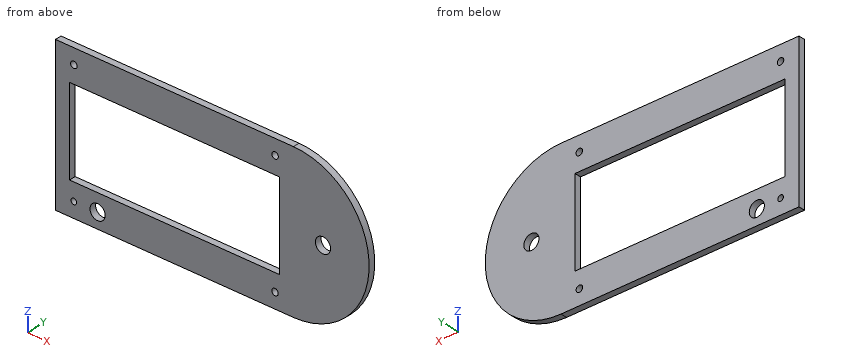
from build123d import *

# Parameters (mm, degrees)
SKETCH1_R           = 1.3
SKETCH1_R_2         = 1.5
SKETCH1_R_3         = 3.5
SKETCH1_W           = 97
SKETCH1_H           = 40
BOSS_EXTRUDE1_DEPTH = 3


with BuildPart() as part:
    # Sketch1 → Boss-Extrude1 (new body)
    with BuildSketch(Plane(origin=(0, 0, 0), x_dir=(1, 0, 0), z_dir=(0, 1, 0))):
        with BuildLine():
            Line((-67.43171984, 21.978952762), (42.56828016, 21.978952762))
            ThreePointArc((42.56828016, 21.978952762), (77.56828016, -13.021047238), (42.56828016, -48.021047238))
            Line((42.56828016, -48.021047238), (-67.43171984, -48.021047238))
            Line((-67.43171984, -48.021047238), (-67.43171984, 21.978952762))
        make_face()
        with Locations((-58.93171984, 14.978952762)):
            Circle(SKETCH1_R, mode=Mode.SUBTRACT)
        with Locations((34.06828016, 14.978952762)):
            Circle(SKETCH1_R_2, mode=Mode.SUBTRACT)
        with Locations((-58.895119552, -41.021035277)):
            Circle(SKETCH1_R_2, mode=Mode.SUBTRACT)
        with Locations((34.104880448, -41.021035277)):
            Circle(SKETCH1_R_2, mode=Mode.SUBTRACT)
        with Locations((56.242935444, -13.021047238)):
            Circle(SKETCH1_R_3, mode=Mode.SUBTRACT)
        with Locations((-47.93171984, 14.978952762)):
            Circle(SKETCH1_R_3, mode=Mode.SUBTRACT)
        with Locations((-12.395119552, -13.021047238)):
            Rectangle(SKETCH1_W, SKETCH1_H, mode=Mode.SUBTRACT)
    extrude(amount=BOSS_EXTRUDE1_DEPTH)


solid = part.part
Input: part model. Units: mm. Frame: model coordinates. Coordinates: 2 decimals unless noted, no trailing zeros. Loops run counter-clockwise (first coordinate to the right, second up) from the corner with the lowest first, then second, coordinate; pieces in that order, holes last.
Q1. Cut plane C-C (y = 1.55). Output: boundary loops of the cut face in (x, z).
Q2. Cut plane B-B (z = 29). Output: boundary loops of the cut face in (x, y).
Q3. Cut plane D-D (x = 68.5). Output: boundary loops of the cut face in (y, z).
Q4. Material intervals for line 1 (Z direction, x = 7, y = 2.6); line 2 (X direction, y = 2.2, z = -15); line 3 (X direction, y = 1, z = 41.5), sorted ascending.
Q5. Cut plane A-A (x = 21). Output: boundary loops of the cut face in (y, z).
Q6. Contact query for flat-ended pins moving along their axis: pin 1 (1.5 mm diameter, centred on y = 1, z = 11.5, fed in from +X); pin 2 (2.5 mm diameter, centred on x = 34.1, z = 41.02, fed in from +Y); pin 3 (1.5 mm diameter, centred on y = 2, z = 18.5, fed in from +X). Output: stop coordinate, or through.
Working result:
1. outline: (-67.43, -21.98) - (42.57, -21.98) arc R35 ccw to (42.57, 48.02) - (-67.43, 48.02) - close; hole (-60.9, -6.98) - (36.1, -6.98) - (36.1, 33.02) - (-60.9, 33.02) - close; hole circle Ø3 at (-58.9, 41.02); hole circle Ø2.6 at (-58.93, -14.98); hole circle Ø7 at (-47.93, -14.98); hole circle Ø3 at (34.07, -14.98); hole circle Ø3 at (34.1, 41.02); hole circle Ø7 at (56.24, 13.02)
2. outline: (-67.43, 0) - (-60.9, 0) - (-60.9, 3) - (-67.43, 3) - close; (36.1, 0) - (73.71, 0) - (73.71, 3) - (36.1, 3) - close
3. outline: (0, -10.49) - (3, -10.49) - (3, 36.53) - (0, 36.53) - close
4. line 1: z = -21.98 to -6.98, 33.02 to 48.02
4. line 2: x = -67.43 to -60.23, -57.63 to -51.43, -44.43 to 32.57, 35.57 to 63.54
4. line 3: x = -67.43 to -60.32, -57.47 to 32.68, 35.53 to 62.91
5. outline: (0, -21.98) - (3, -21.98) - (3, -6.98) - (0, -6.98) - close; (0, 33.02) - (3, 33.02) - (3, 48.02) - (0, 48.02) - close
6. pin 1: stops at x = 77.56
6. pin 2: passes through
6. pin 3: stops at x = 77.25
